Check sheet for the drawn part. Datum: minimum x, y, z corner. Units: mm. A direction names the side the tool comes from. Round coordinates to 2 decimals unless told otherwise and drop trailing zeros. Order: outer loops, then holes, each group sorted by start corner. A loop starts at its lowest first (then second) coordinate and runs counter-clockwise, first axis right, second up.
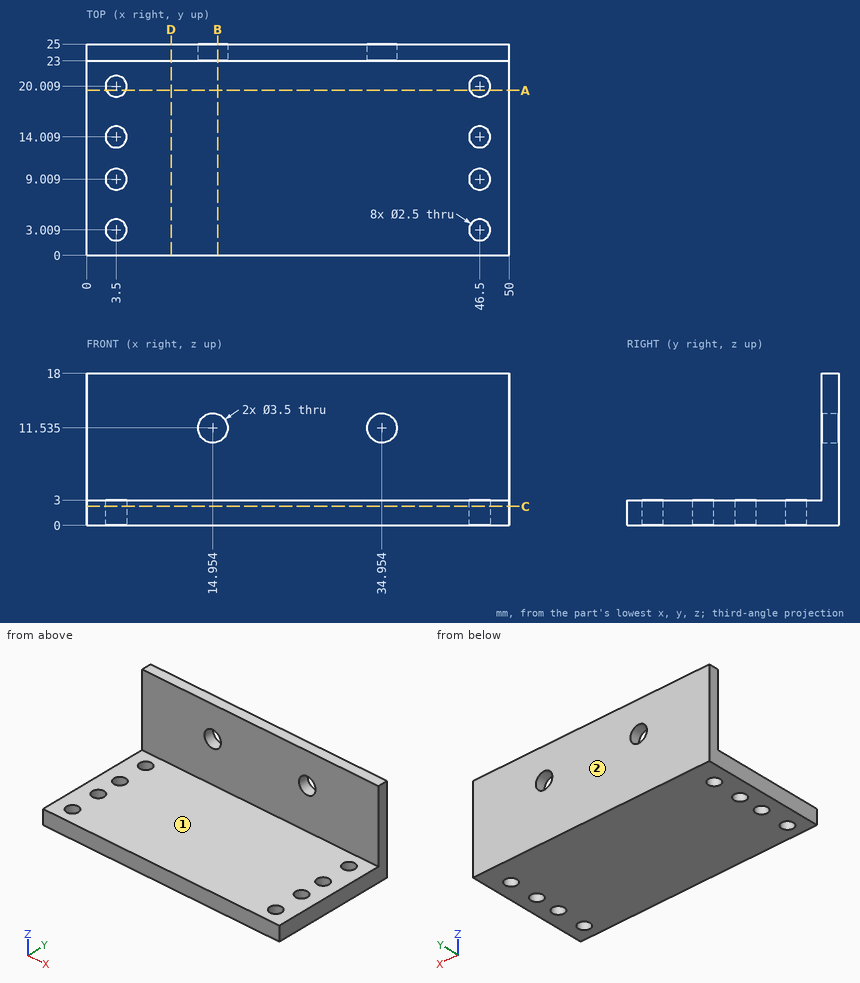
(1) Sectioned sample at B-B, the plane x = 15.5. Record the cut outline in (y, z).
Returned:
outline: (0, 0) - (25, 0) - (25, 9.87) - (23, 9.87) - (23, 3) - (0, 3) - close; (23, 13.2) - (25, 13.2) - (25, 18) - (23, 18) - close
(2) Set-up check for the marked faces 1 and 2: record each of +Z, -Z, +X, -X, +Y, -Y from which the full face is reachable in a straight line by a thin tool's end or side.
Returned:
face 1: +Z, +X, -X, -Y
face 2: +Z, -Z, +X, -X, +Y
(3) Sectioned sample at C-C, the plane z = 2.25. Give the number of separate pieces and of enclosed holes in the cut face, and give its area (3 significant figures).
Returned:
separate pieces: 1
enclosed holes: 8
area: 1,210 mm2
(4) Material ranges on line 1 (Z direction, x = 18.5, y = 4.25); line 2 (Y direction, x = 40.5, z = 16.25), recorded low to high.
Returned:
line 1: z = 0 to 3
line 2: y = 23 to 25
(5) Sectioned sample at A-A, the plane y = 19.5. Record the cut outline in (x, z).
Returned:
outline: (0, 0) - (2.36, 0) - (2.36, 3) - (0, 3) - close; (4.64, 0) - (45.36, 0) - (45.36, 3) - (4.64, 3) - close; (47.64, 0) - (50, 0) - (50, 3) - (47.64, 3) - close
(6) Depth check by flat-ended pin: P1, Ø3, axis at x = 34.95, z = 11.54, coming from the -Y side; P2, Ø11.5, axis at x = 29.5, y = 11.5, coming from the +Z side; P3, Ø7.5, axis at x = 19, z = 10, coming from the -Y side. Enter the tip coordinate at first touch or a pass-through.
Returned:
P1: passes through
P2: stops at z = 3
P3: stops at y = 23
(7) Sectioned sample at D-D, the plane x = 10. Record the cut outline in (y, z), and give its area (3 significant figures).
Returned:
outline: (0, 0) - (25, 0) - (25, 18) - (23, 18) - (23, 3) - (0, 3) - close
area: 105 mm2
